Drawing for the job (mm, zero at the part's lowest x, y, z). Give positions to 0.01 mm unless a question says otherwise; leave off trailing zeros. Loops run counter-clockwise (first coordinate to the right, second up) from the corner with the lowest first, then second, coordinate; pieces in that order, holes last.
1) Two-plate mould, pull along Z, no slides. Class the marked faces 1 and 2: +Z half, -Z half, draft (parallel to the pull), parting line (faces both ways), or undercut.
2) Wall check: line 1 (Z direction, x = 46, y = 5.5); line 2 (Z direction, x = 8.5, y = 3.25); line 3 (Y direction, x = 15.5, z = 0.8). Give the ranges that are in metal, low to high.
3) Band-saw the part on A-A on x = 41.5. List the corners of the cut face in (y, z).
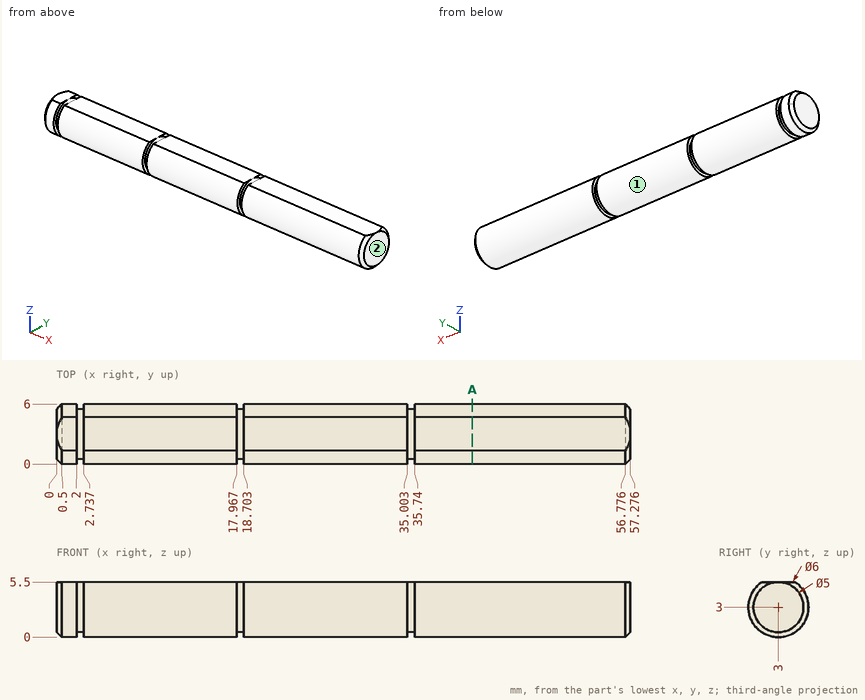
Findings below:
1. face 1: parting line
1. face 2: draft
2. line 1: z = 1.34 to 4.66
2. line 2: z = 0.01 to 5.5
2. line 3: y = 0.96 to 5.04
3. outline: (1.34, 5.5) arc R3 ccw (long way) to (4.66, 5.5) - close
